from build123d import *

# Parameters (mm, degrees)
F1_DEPTH = 50.8
F3_W     = 17.0859034664
F3_H     = 221.488
F4_DEPTH = 25.4
F8_DEPTH = 508.508


with BuildPart() as f1:
    # F0 (on Top) → F1 (new body)
    with BuildSketch(Plane.XY):
        Polygon((0, -261.7343), (0, 261.7343), (-156.1992195996, 0), align=None)
    extrude(amount=F1_DEPTH)

    # F3 (on offset) → F4 (join)
    with BuildSketch(Plane.XY.offset(50.8)):
        with Locations((-8.5429517332, -7.1447751335)):
            Rectangle(F3_W, F3_H)
        Polygon((-42.5371713936, -13.3966989815), (-23.862991482, -13.3966989815), (-23.862991482, 13.3966989815), (-42.5371713936, 13.3966989815), (-61.2113513052, 13.3966989815), (-61.2113513052, 0), (-61.2113513052, -13.3966989815), align=None)
        Polygon((-59.9951921275, -116.2100359797), (-42.5371713936, -13.3966989815), (-61.2113513052, -13.3966989815), (-61.2113513052, 0), (-85.2522104979, -116.2100359797), align=None)
        Polygon((-61.2113513052, 13.3966989815), (-42.5371713936, 13.3966989815), (-64.5063391738, 103.6467850208), (-92.7901566029, 103.6467850208), (-61.2113513052, 0), align=None)
    extrude(amount=F4_DEPTH)

    # F7 (on offset) → F8 (join)
    with BuildSketch(Plane.XZ.offset(246.38)):
        Polygon((0, 30.5890981108), (0, 20.4187799245), (6.6587165929, 12.7179827541), (6.6587165929, 38.0452573299), align=None)
    extrude(amount=-F8_DEPTH)


solid = f1.part
Geometry: final body of the model. Coordinates: model frame, mm. A direction names the side the tool comes from. Coordinates: 2 decimals unless noted, no trailing zeros. Order: outer loops, then holes, each group sorted by start corner. A loop starts at its lowest first (then second) coordinate and runs counter-clockwise, first axis right, second up.
(1) Section query D-D (y = -99). Return the cut outline in (x, z), plus the area to 3 significant figures.
(2) Section query A-A (y = -199.5). Return the cut outline in (x, z).
(3) First-contact query: pin 1 (5.5 mm diameter, centred on x = -35.5, z = 62.5, fed in from -Y); pin 2 (1.5 mm diameter, centred on y = -29.5, z = 30, fed in from -X); pin 3 (3 mm diameter, centred on y = 193, z = 33, fed in from -X). Flat tips, straight axial feed; report the tip coordinate or a pass-through.
(4) Section query C-C (x = -109). Return the cut outline in (y, z).
(5) Draft query along X for faces 1 (the face through (0, -4, 38)), 2 (the face through (-53.37, 57.89, 63.32)), 3 (the face through (-9, -117.889, 63)), 4 (the face through (-77.006, 132.699, 25.044)). Return one class per face: pulls with the +X half, pulls with the -X half, needs draft (parallel to the pull), parting line crosses it, or undercut.
(6) Material intervals for probe 1 along Z at (x, y) = (-123, -37); probe 2 along X at (y, z) = (-33.5, 66.5); probe 3 along Y at (x, z) = (-25, 60), sorted ascending.
(7) Section query B-B (z = 46). Return the cut outline in (x, y), plus the area to 3 significant figures.
(8) Access query for faces 5 (the face through (-23.863, 0, 63)), 6 (the face through (-73, -116.21, 63)), 7 (the face through (-9, 103.599, 63)), 8 (the face through (-77.222, 52.549, 63.322)), 9 (the face through (-33, -13.397, 63)). Directions: +Z, -Z, +X, -X, +Y, -Y. A direction counts if a zero-diameter tool reaches every point of the face in a straight line with its end or side. Return the directions, or none.
Solution:
1. outline: (-97.12, 0) - (0, 0) - (0, 20.42) - (6.66, 12.72) - (6.66, 38.05) - (0, 30.59) - (0, 76.2) - (-17.09, 76.2) - (-17.09, 50.8) - (-57.07, 50.8) - (-57.07, 76.2) - (-81.69, 76.2) - (-81.69, 50.8) - (-97.12, 50.8) - close
1. area: 6,110 mm2
2. outline: (-37.14, 0) - (0, 0) - (0, 20.42) - (6.66, 12.72) - (6.66, 38.05) - (0, 30.59) - (0, 50.8) - (-37.14, 50.8) - close
3. pin 1: stops at y = -13.4
3. pin 2: stops at x = -139.04
3. pin 3: stops at x = -41.91
4. outline: (-79.09, 0) - (79.09, 0) - (79.09, 50.8) - (-79.09, 50.8) - close
5. face 1: undercut
5. face 2: undercut
5. face 3: needs draft
5. face 4: pulls with the -X half
6. probe 1: z = 0 to 50.8
6. probe 2: x = -68.14 to -45.95, -17.09 to 0
6. probe 3: y = -13.4 to 13.4
7. outline: (-156.2, 0) - (0, -261.73) - (0, 261.73) - close
7. area: 40,900 mm2
8. face 5: +Z, +Y, -Y
8. face 6: +Z, -X, -Y
8. face 7: +Z, +X, -X, +Y
8. face 8: +Z, -X
8. face 9: +Z, -Y
